```python
from build123d import *

# Parameters (mm, degrees)
BOSS_EXTRUDE1_DEPTH = 5.715


with BuildPart() as part:
    # Model → Boss-Extrude1 (new body)
    with BuildSketch(Plane.XY):
        Polygon((544.68776, 28.91536), (549.67378, 28.91536), (549.67378, 23.2006394), (561.10632, 23.2006394), (561.10632, 28.91536), (572.53378, 28.91536), (572.53378, 23.2006394), (583.96378, 23.2006394), (583.96378, 28.91536), (595.39378, 28.91536), (595.39378, 23.2006394), (606.82378, 23.2006394), (606.82378, 28.91536), (618.25632, 28.91536), (618.25632, 23.2006394), (629.68378, 23.2006394), (629.68378, 28.91536), (641.11378, 28.91536), (641.11378, 23.2006394), (652.54378, 23.2006394), (652.54378, 28.91536), (663.97378, 28.91536), (663.97378, 23.2006394), (675.40632, 23.2006394), (675.40632, 28.91536), (686.83378, 28.91536), (686.83378, 23.2006394), (698.26378, 23.2006394), (698.26378, 28.91536), (709.69378, 28.91536), (709.69378, 23.2006394), (721.12378, 23.2006394), (721.12378, 28.91536), (732.55632, 28.91536), (732.55632, 23.2006394), (743.98378, 23.2006394), (743.98378, 28.91536), (755.41378, 28.91536), (755.41378, 23.2006394), (766.84378, 23.2006394), (766.84378, 28.91536), (778.27378, 28.91536), (778.27378, 23.2006394), (789.70632, 23.2006394), (789.70632, 28.91536), (794.68726, 28.91536), (794.68726, 42.83075), (800.40226, 42.83075), (800.40226, 54.260496), (794.68726, 54.260496), (794.68726, 65.691004), (800.40226, 65.691004), (800.40226, 77.120496), (794.68726, 77.120496), (794.68726, 88.549988), (800.40226, 88.549988), (800.40226, 99.98075), (794.68726, 99.98075), (794.68726, 111.410496), (800.40226, 111.410496), (800.40226, 122.841004), (794.68726, 122.841004), (794.68726, 134.270496), (800.40226, 134.270496), (800.40226, 145.699988), (794.68726, 145.699988), (794.68726, 157.13075), (800.40226, 157.13075), (800.40226, 168.560496), (794.68726, 168.560496), (794.68726, 179.991004), (800.40226, 179.991004), (800.40226, 191.420496), (794.68726, 191.420496), (794.68726, 202.849988), (800.40226, 202.849988), (800.40226, 214.28075), (794.68726, 214.28075), (794.68726, 225.710496), (800.40226, 225.710496), (800.40226, 237.141004), (794.68726, 237.141004), (794.68726, 248.570496), (800.40226, 248.570496), (800.40226, 259.99948), (794.68726, 259.99948), (794.68726, 273.91614), (789.70632, 273.91614), (789.70632, 279.63114), (778.27378, 279.63114), (778.27378, 273.91614), (766.84378, 273.91614), (766.84378, 279.63114), (755.41378, 279.63114), (755.41378, 273.91614), (743.98378, 273.91614), (743.98378, 279.63114), (732.55632, 279.63114), (732.55632, 273.91614), (721.12378, 273.91614), (721.12378, 279.63114), (709.69378, 279.63114), (709.69378, 273.91614), (698.26378, 273.91614), (698.26378, 279.63114), (686.83378, 279.63114), (686.83378, 273.91614), (675.40632, 273.91614), (675.40632, 279.63114), (663.97378, 279.63114), (663.97378, 273.91614), (652.54378, 273.91614), (652.54378, 279.63114), (641.11378, 279.63114), (641.11378, 273.91614), (629.68378, 273.91614), (629.68378, 279.63114), (618.25632, 279.63114), (618.25632, 273.91614), (606.82378, 273.91614), (606.82378, 279.63114), (595.39378, 279.63114), (595.39378, 273.91614), (583.96378, 273.91614), (583.96378, 279.63114), (572.53378, 279.63114), (572.53378, 273.91614), (561.10632, 273.91614), (561.10632, 279.63114), (549.67378, 279.63114), (549.67378, 273.91614), (544.68776, 273.91614), (544.68776, 259.99948), (538.97276, 259.99948), (538.97276, 248.570496), (544.68776, 248.570496), (544.68776, 237.141004), (538.97276, 237.141004), (538.97276, 225.710496), (544.68776, 225.710496), (544.68776, 214.28075), (538.97276, 214.28075), (538.97276, 202.849988), (544.68776, 202.849988), (544.68776, 191.420496), (538.97276, 191.420496), (538.97276, 179.991004), (544.68776, 179.991004), (544.68776, 168.560496), (538.97276, 168.560496), (538.97276, 157.13075), (544.68776, 157.13075), (544.68776, 145.699988), (538.97276, 145.699988), (538.97276, 134.270496), (544.68776, 134.270496), (544.68776, 122.841004), (538.97276, 122.841004), (538.97276, 111.410496), (544.68776, 111.410496), (544.68776, 99.98075), (538.97276, 99.98075), (538.97276, 88.549988), (544.68776, 88.549988), (544.68776, 77.120496), (538.97276, 77.120496), (538.97276, 65.691004), (544.68776, 65.691004), (544.68776, 54.260496), (538.97276, 54.260496), (538.97276, 42.83075), (544.68776, 42.83075), align=None)
    extrude(amount=BOSS_EXTRUDE1_DEPTH)


solid = part.part
```
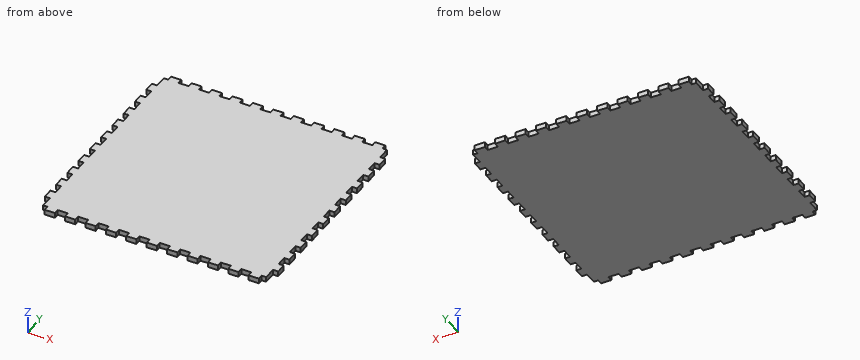
Here's how the part is built. I have some questions about the finished solid (model axes, mm). Coordinates: 2 decimals unless noted, no trailing zeros. Write each loop counter-clockwise with the first axis right and the second up, starting at its lowest first coordinate (ties: lowest second). Pieces come first, ordered by that corner, then holes. Notation, with made-up numbers: (36.5, -26.75) -> (40.5, -26.75) arc R27 ccw to (40.5, -6.75) -> close; hole circle Ø7 at (18.5, -2). An arc over 180 degrees is marked (long way). Use a Markdown table: item, result. Add a question column.
(1) If we section it at B-B, the plane x = 637: Write out the boundary of the cut face in (y, z) (3 decimals).
(2) Please list where these lines run through material, in increasing order: line 1 (X direction, y = 35.5, z = 4.3); line 2 (Y direction, x = 728, z = 2.85).
(3) I'm going to push flat-ended pins straight in: P1, Ø3, axis at x = 733, y = 220, coming from the -Z side; P2, Ø1.7, axis at y = 25.5, z = 2, coming from the +X side; P3, Ø1.7, axis at x = 541, z = 3, coming from the -Y side; P4, Ø3, axis at x = 796.5, z = 3.5, coming from the +Y side. Where does each tip first touch, or does it pass through?
(4) If we section it at A-A, the plane y = 197: Write out the boundary of the cut face in (x, z) (3 decimals), and give its area (3 significant figures).
Outcome:
| question | item | result |
|---|---|---|
| 1 | outline | (28.915, 0) -> (273.916, 0) -> (273.916, 5.715) -> (28.915, 5.715) -> close |
| 2 | line 1 | x = 544.69 to 794.69 |
| 2 | line 2 | y = 28.92 to 273.92 |
| 3 | P1 | stops at z = 0 |
| 3 | P2 | stops at x = 789.71 |
| 3 | P3 | stops at y = 42.83 |
| 3 | P4 | stops at y = 260 |
| 4 | outline | (544.688, 0) -> (794.687, 0) -> (794.687, 5.715) -> (544.688, 5.715) -> close |
| 4 | area | 1,430 mm^2 |
